```python
from build123d import *

# Parameters (mm, degrees)
BOSS_EXTRUDE5_DEPTH = 15
BOSS_EXTRUDE6_DEPTH = 5
SKETCH3_W           = 2
SKETCH3_H           = 39.156418696
CUT_EXTRUDE1_DEPTH  = 10
FILLET2_R           = 1


with BuildPart() as part:
    # Sketch2 → Boss-Extrude5 (new body)
    with BuildSketch(Plane.XY.offset(5)):
        with BuildLine():
            Line((-14.5, 19.421790652), (14.5, 19.421790652))
            add(Edge.make_bspline(
                [(14.5, 19.421790652), (34.327554894, 15.095349213), (48, 10.176108588)],
                knots=[0, 0, 0, 1, 1, 1], degree=2))
            Line((48, 10.176108588), (48, -19.578209348))
            Line((48, -19.578209348), (-48, -19.578209348))
            Line((-48, -19.578209348), (-48, 10.176108588))
            add(Edge.make_bspline(
                [(-14.5, 19.421790652), (-34.327554894, 15.095349213), (-48, 10.176108588)],
                knots=[0, 0, 0, 1, 1, 1], degree=2))
        make_face()
    extrude(amount=BOSS_EXTRUDE5_DEPTH)

    # Sketch1 → Boss-Extrude6 (add)
    # profile 1 of 2: a face of its own
    with BuildSketch(Plane.XY):
        with BuildLine():
            Line((-15, 21.421790652), (-34.887462632, 16.495927254))
            ThreePointArc((-34.887462632, 16.495927254), (-39.255473059, 16.793838072), (-42.632407856, 19.580337189))
            ThreePointArc((-42.632407856, 19.580337189), (-47.124640259, 21.2604342), (-50, 17.421790652))
            Line((-50, 17.421790652), (-50, -21.578209348))
            Line((-50, -21.578209348), (50, -21.578209348))
            Line((50, -21.578209348), (50, 17.421790652))
            ThreePointArc((50, 17.421790652), (47.124640259, 21.2604342), (42.632407856, 19.580337189))
            ThreePointArc((42.632407856, 19.580337189), (39.255473059, 16.793838072), (34.887462632, 16.495927254))
            Line((34.887462632, 16.495927254), (15, 21.421790652))
            Line((15, 21.421790652), (-15, 21.421790652))
        make_face()
        with BuildLine():
            add(Edge.make_bspline(
                [(-14.5, 19.421790652), (-34.327554894, 15.095349213), (-48, 10.176108588)],
                knots=[0, 0, 0, 1, 1, 1], degree=2))
            Line((-48, 10.176108588), (-48, -19.578209348))
            Line((-48, -19.578209348), (48, -19.578209348))
            Line((48, -19.578209348), (48, 10.176108588))
            add(Edge.make_bspline(
                [(14.5, 19.421790652), (34.327554894, 15.095349213), (48, 10.176108588)],
                knots=[0, 0, 0, 1, 1, 1], degree=2))
            Line((14.5, 19.421790652), (-14.5, 19.421790652))
        make_face(mode=Mode.SUBTRACT)
    # profile 2 of 2: a face of its own
    with BuildSketch(Plane.XY):
        with BuildLine():
            Line((-14.5, 19.421790652), (14.5, 19.421790652))
            add(Edge.make_bspline(
                [(14.5, 19.421790652), (34.327554894, 15.095349213), (48, 10.176108588)],
                knots=[0, 0, 0, 1, 1, 1], degree=2))
            Line((48, 10.176108588), (48, -19.578209348))
            Line((48, -19.578209348), (-48, -19.578209348))
            Line((-48, -19.578209348), (-48, 10.176108588))
            add(Edge.make_bspline(
                [(-14.5, 19.421790652), (-34.327554894, 15.095349213), (-48, 10.176108588)],
                knots=[0, 0, 0, 1, 1, 1], degree=2))
        make_face()
    extrude(amount=BOSS_EXTRUDE6_DEPTH)

    # Sketch3 → Cut-Extrude1 (cut)
    with BuildSketch(Plane.XY.offset(20)):
        Rectangle(SKETCH3_W, SKETCH3_H)
    extrude(amount=-CUT_EXTRUDE1_DEPTH, mode=Mode.SUBTRACT)

    # Fillet2
    fillet2_edges = [part.edges().sort_by_distance(p)[0] for p in [
        (1, -0.078209348, 10),
        (-1, -0.078209348, 10),
    ]]
    fillet(fillet2_edges, radius=FILLET2_R - 0.0001)  # a hair under: the kernel refuses the full size


solid = part.part
```
Check sheet for the modelled part. Datum: model origin and axes. Units: mm. A direction names the side the tool comes from. Round coordinates to 2 decimals unless told otherwise and drop trailing zeros. Order: outer loops, then holes, each group sorted by start corner. A loop starts at its lowest first (then second) coordinate and runs counter-clockwise, first axis right, second up. Notation, with made-up numbers: M 28.5,59.25 L 34.5,59.25 A30 ccw 34.5,90.25 Z; hole C 69,29 d7. An arc over 180 degrees is marked long. Answer in a Markdown table with one row per item.
(1) Draft check along X on faces 1 (the flat face through (-24.805, 18.993, 2.465)), 2 (the flat face through (-24, 0, 20)), 3 (the cylindrical face through (39.313, 16.817, 2.465)), 4 (the flat face through (50, -2, 2)). Enter one of: +X half, -X half, draft (parallel to the pull), parting line (faces both ways), or undercut.
Findings:
| item | result |
|---|---|
| face 1 | undercut |
| face 2 | draft |
| face 3 | undercut |
| face 4 | +X half |
(2) Material ranges on line 1 along X through (y, z) = (-11.5, 13.25); line 2 along Y through (x, z) = (-12.5, 13.75); line 3 along X through (y, z) = (7.5, 10.5), recorded low to high. Write a range as from..to.
Findings:
| item | result |
|---|---|
| line 1 | x = -48..-1, 1..48 |
| line 2 | y = -19.58..19.42 |
| line 3 | x = -48..-0.87, 0.87..48 |
(3) Section check B-B on x = -3.5. Record the boundary of the cut face in (y, z), plus the area to 3 significant figures.
Findings:
| item | result |
|---|---|
| outline | M -21.58,0 L 21.42,0 L 21.42,5 L 19.42,5 L 19.42,20 L -19.58,20 L -19.58,5 L -21.58,5 Z |
| area | 800 mm^2 |
(4) Gauge pin test, flat ends, axial feed: pin 1 (7.5 mm diameter, centred on y = -7, z = 11.5, fed in from +X); pin 2 (4.5 mm diameter, centred on x = -3.5, z = 10.5, fed in from +Y); pin 3 (4.5 mm diameter, centred on y = -9.5, z = 15, fed in from -X). Record the tip position at first contact, or that the pin passes through.
Findings:
| item | result |
|---|---|
| pin 1 | stops at x = 48 |
| pin 2 | stops at y = 19.42 |
| pin 3 | stops at x = -48 |
(5) Set-up check for faces 5 (the flat face through (1, -19.578, 9)), 6 (the flat face through (0, 19.422, 9)), 7 (the flat face through (25.083, 18.924, 2.465)), 8 (the flat face through (48, -4, 12)), 9 (the flat face through (1, 0, 16)): record each of +Z, -Z, +X, -X, +Y, -Y from which the full face is reachable in a straight line by a thin tool's end or side.
Findings:
| item | result |
|---|---|
| face 5 | +Z, +X, -X, -Y |
| face 6 | +Z, +X, -X, +Y |
| face 7 | +Z, -Z, +Y |
| face 8 | +Z, +X, +Y, -Y |
| face 9 | +Z, +Y, -Y |
